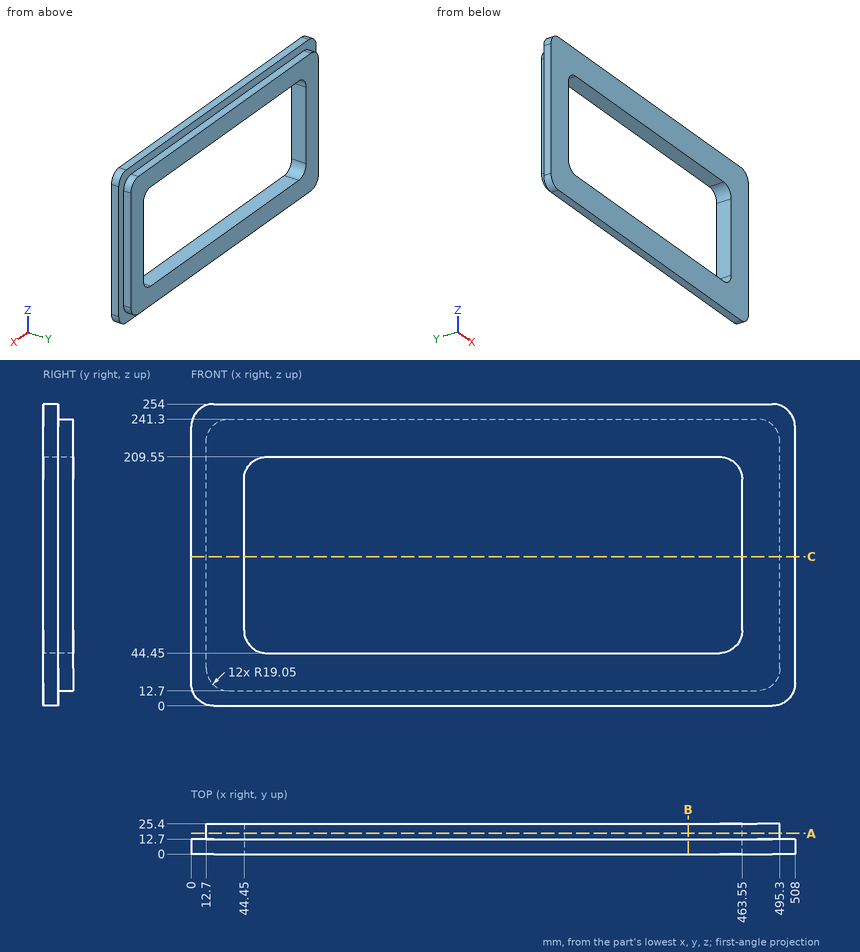
Check sheet for the drawn part. Datum: minimum x, y, z corner. Units: mm. Round coordinates to 2 decimals unless told otherwise and drop trailing zeros. Loops run counter-clockwise (first coordinate to the right, second up) from the corner with the lowest first, then second, coordinate; pieces in that order, holes last. Notation, with made-up numbers: (49, 76.5) - (73, 76.5) arc R25 cw to (73, 109.5) - close; hole circle Ø10 at (10.5, -10.5). An arc over 180 degrees is marked (long way). Answer as a JSON object with one key per item and string values. Group by question number.
Q1. Sectioned sample at C-C, the plane z = 125.5. Enter the section's corners in (x, y).
Q2. Scan lines: line 1 along Z through (x, y) = (91, 1.75); line 2 along X through (y, z) = (1, 129); line 3 along Z through (x, y) = (151, 16). Record each from-to range of solid material in increasing order. Write a range as [from, to].
Q3. Gauge pin test, flat ends, axial feed: P1, Ø6, axis at x = 292.5, y = 18, coming from the +Z side; P2, Ø4, axis at x = 270.5, y = 19, coming from the -Z side; P3, Ø10, axis at y = 21, z = 162.5, coming from the -X side. Record the tip position at first contact, or that the pin passes through.
Q4. Sectioned sample at B-B, the plane x = 418. Enter the section's corners in (y, z), plus the area to 3 significant figures.
Q5. Sectioned sample at A-A, the plane y = 17.5. Enter the section's corners in (x, z), plus the area to 3 significant figures.
Solution:
{
 "1": {"outline": "(0, 0) - (44.45, 0) - (44.45, 25.4) - (12.7, 25.4) - (12.7, 12.7) - (0, 12.7) - close; (463.55, 0) - (508, 0) - (508, 12.7) - (495.3, 12.7) - (495.3, 25.4) - (463.55, 25.4) - close"},
 "2": {"line 1": "z = [0, 44.45], [209.55, 254]", "line 2": "x = [0, 44.45], [463.55, 508]", "line 3": "z = [12.7, 44.45], [209.55, 241.3]"},
 "3": {"P1": "stops at z = 241.3", "P2": "stops at z = 12.7", "P3": "stops at x = 12.7"},
 "4": {"outline": "(0, 0) - (12.7, 0) - (12.7, 12.7) - (25.4, 12.7) - (25.4, 44.45) - (0, 44.45) - close; (0, 209.55) - (25.4, 209.55) - (25.4, 241.3) - (12.7, 241.3) - (12.7, 254) - (0, 254) - close", "area": "1,940 mm²"},
 "5": {"outline": "(12.7, 31.75) arc R19.05 ccw to (31.75, 12.7) - (476.25, 12.7) arc R19.05 ccw to (495.3, 31.75) - (495.3, 222.25) arc R19.05 ccw to (476.25, 241.3) - (31.75, 241.3) arc R19.05 ccw to (12.7, 222.25) - close; hole (44.45, 63.5) arc R19.05 ccw to (63.5, 44.45) - (444.5, 44.45) arc R19.05 ccw to (463.55, 63.5) - (463.55, 190.5) arc R19.05 ccw to (444.5, 209.55) - (63.5, 209.55) arc R19.05 ccw to (44.45, 190.5) - close", "area": "41,100 mm²"}
}
